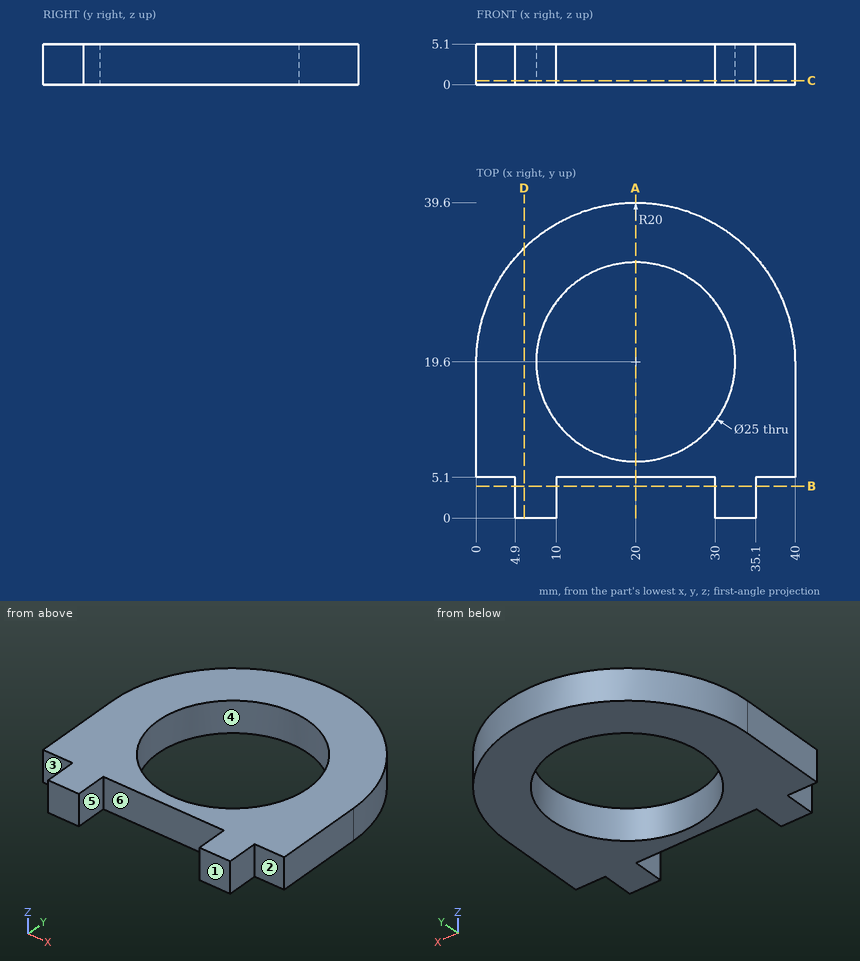
For this review, use the dimensioned drawing (mm, ordinates from the lowest corner) and the shaded views. A direction names the side the tool comes from. Round coordinates to 2 decimals unless told otherwise and drop trailing zeros. Loops run counter-clockwise (first coordinate to the right, second up) from the corner with the lowest first, then second, coordinate; pieces in that order, holes last. Notation, with made-up numbers: (65.5, 24) -> (115.5, 24) arc R21 cw to (115.5, 54) -> close; hole circle Ø5 at (8, -6). An arc over 180 degrees is marked (long way). Write item = value, one per line. Start each with the question number.
Item 1: For the marked faces 1, 2 and 3, list the 3-axis set-ups (+Z, -Z, +X, -X, +Y, -Y) from which the entire face can be reached by the end or side of a thin tool; tool diameter is ignored.
Item 2: Take a section at B-B on y = 4. Give the boundary of the cut face in (x, z).
Item 3: Mouldability with a two-part tool opening along Y and no side actions: class the marked faces 4, 5 and 6 as released by +Y, released by -Y, zero draft, split by the parting line, or undercut.
Item 4: Take a section at C-C on z = 0.5. Give the boundary of the cut face in (x, y).
Item 5: To check wall thickness, follow L1, parallel to Y at x = 20, z = 2.3; L2, parallel to X at y = 5, z = 0.5; L3, parallel to X at y = 25.5, z = 2.4. State the ranges of each line that lie inside material, in increasing order.
Item 6: Take a section at D-D on x = 6. Give the boundary of the cut face in (y, z).
Item 7: Insertion check: pin 1 (2.5 mm diameter, centred on y = 3.5, z = 1.5, fed in from +X); pin 2 (1.5 mm diameter, centred on x = 25.5, z = 1, fed in from +Y); pin 3 (1.5 mm diameter, centred on x = 38.5, z = 3, fed in from -Y). Each pin has a flat end and moves straight along its axis. Give the tip position at first contact, or say it passes through.
Item 8: Take a section at A-A on x = 20. Give the boundary of the cut face in (y, z), plus the area to 4 significant figures.
Result:
q1.face_1 = +Z, -Z, +X, -X, -Y
q1.face_2 = +Z, -Z, +X, -Y
q1.face_3 = +Z, -Z, -X, -Y
q2.outline = (4.9, 0) -> (10, 0) -> (10, 5.1) -> (4.9, 5.1) -> close; (30, 0) -> (35.1, 0) -> (35.1, 5.1) -> (30, 5.1) -> close
q3.face_4 = undercut
q3.face_5 = zero draft
q3.face_6 = released by -Y
q4.outline = (0, 5.1) -> (4.9, 5.1) -> (4.9, 0) -> (10, 0) -> (10, 5.1) -> (30, 5.1) -> (30, 0) -> (35.1, 0) -> (35.1, 5.1) -> (40, 5.1) -> (40, 19.6) arc R20 ccw to (0, 19.6) -> close; hole circle Ø25 at (20, 19.6)
q5.L1 = 5.1 to 7.1, 32.1 to 39.6
q5.L2 = 4.9 to 10, 30 to 35.1
q5.L3 = 0.89 to 8.98, 31.02 to 39.11
q6.outline = (0, 0) -> (33.88, 0) -> (33.88, 5.1) -> (0, 5.1) -> close
q7.pin_1 = 35.1
q7.pin_2 = 39.03
q7.pin_3 = 5.1
q8.outline = (5.1, 0) -> (7.1, 0) -> (7.1, 5.1) -> (5.1, 5.1) -> close; (32.1, 0) -> (39.6, 0) -> (39.6, 5.1) -> (32.1, 5.1) -> close
q8.area = 48.45 mm²
